Design review of the part built by this model. Coordinates are the model's own, in mm. Face numbers are marked on the shaded views. A direction names the side the tool comes from. Coordinates: 2 decimals unless noted, no trailing zeros. Loops run counter-clockwise (first coordinate to the right, second up) from the corner with the lowest first, then second, coordinate; pieces in that order, holes last. Notation, with made-up numbers: M 21.25,16.25 L 43.25,16.25 A23 cw 43.25,29.25 Z; hole C 22.25,-20.75 d8. An arc over 180 degrees is marked long. One line per item, written item: value.
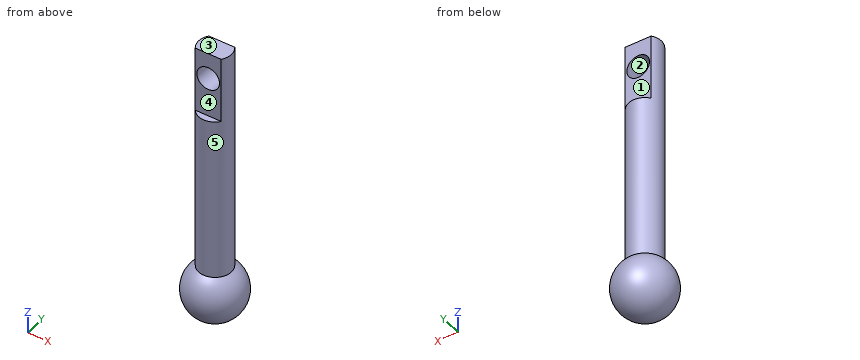
```python
from build123d import *

# Parameters (mm, degrees)
CUT_EXTRUDE3_START      = -10
CUT_EXTRUDE3_DEPTH      = 10
CUT_EXTRUDE4_DEPTH      = 44.707447118
CUT_EXTRUDE4_DEPTH_BACK = 44.707447118
SKETCH4_R               = 1.75


with BuildPart() as part:
    # Sketch1 → Revolve1 (revolve)
    with BuildSketch(Plane(origin=(0, 0, 0), x_dir=(1, 0, 0), z_dir=(0, 1, 0)), mode=Mode.PRIVATE) as revolve1_sk:
        with BuildLine():
            Line((0, 43.241657387), (0, 0))
            Line((0, 0), (2.5, 0))
            Line((2.5, 0), (2.5, 35))
            ThreePointArc((2.5, 35), (4.30624304, 40.047900427), (0, 43.241657387))
        make_face()
    revolve(revolve1_sk.sketch.rotate(Axis((0, 0, -43.241657387), (0, 0, 1)), 180), axis=Axis((0, 0, -43.241657387), (0, 0, 1)))

    # Sketch2 → Cut-Extrude3 (cut)
    with BuildSketch(Plane.XY.offset(CUT_EXTRUDE3_START)):
        with BuildLine():
            ThreePointArc((2, 1.5), (0, 2.5), (-2, 1.5))
            Line((-2, 1.5), (2, 1.5))
        make_face()
        with BuildLine():
            Line((2, -1.5), (-2, -1.5))
            ThreePointArc((-2, -1.5), (0, -2.5), (2, -1.5))
        make_face()
    extrude(amount=CUT_EXTRUDE3_DEPTH, mode=Mode.SUBTRACT)

    # Sketch4 → Cut-Extrude4 (cut, two sides: drawn at the far end of the back side and taken through both)
    with BuildSketch(Plane(origin=(0, 0, 0), x_dir=(1, 0, 0), z_dir=(0, 1, 0)).offset(-CUT_EXTRUDE4_DEPTH_BACK)):
        with Locations(Location((0, 4, 0), (0, 0, 90))):
            Circle(SKETCH4_R)
    extrude(amount=CUT_EXTRUDE4_DEPTH + CUT_EXTRUDE4_DEPTH_BACK, mode=Mode.SUBTRACT)


solid = part.part
```
(1) We need section D-D on z = -26. State the section outline as (x, y) points, then the cut area to 3 significant figures.
Reply:
outline: C 0,0 d5
area: 19.6 mm2
(2) We need section B-B on y = 0. State the section outline as (x, z) points, then the cut area to 3 significant figures.
Reply:
outline: M -2.5,-35 A4.5 ccw long 2.5,-35 L 2.5,0 L -2.5,0 Z; hole C 0,-4 d3.5
area: 226 mm2
(3) Insertion check: pin 1 (1 mm diameter, centred on x = -2, y = -2.5, fed in from -Z); pin 2 (5 mm diameter, centred on x = 3, z = -17, fed in from -Y); pin 3 (5 mm diameter, centred on x = -1.5, z = -28, fed in from +Y). Each pin has a flat end and moves straight along its axis. Give the tip position at first contact, or say it passes through.
Reply:
pin 1: stops at z = -42.34
pin 2: stops at y = -2.45
pin 3: stops at y = 2.5
(4) Tool access review of the marked faces 4 and 5: name each direction out of +Z, -Z, +X, -X, +Y, -Y from which nothing blocks a thin tool from reaching the whole face with its end or side.
Reply:
face 4: +Z, +X, -X, -Y
face 5: +Z
(5) We need section A-A on z = -4. State the section outline as (x, y) points.
Reply:
outline: M -2,-1.5 L -1.75,-1.5 L -1.75,1.5 L -2,1.5 A2.5 ccw Z; M 1.75,-1.5 L 2,-1.5 A2.5 ccw 2,1.5 L 1.75,1.5 Z
(6) Mouldability with a two-part tool opening along Z and no side actions: class the marked faces 1, 2 and 3 as released by +Z, released by -Z, zero draft, split by the parting line, or undercut.
Reply:
face 1: zero draft
face 2: undercut
face 3: released by +Z
(7) To check wall thickness, follow line 1 along X through (y, z) = (0.1, -4); line 2 along Y through (x, z) = (-0.5, -1.5); line 3 along Z through (x, y) = (0.25, 0). State the ranges of each line that lie inside material, in increasing order. Write a range as [from, to].
Reply:
line 1: x = [-2.5, -1.75], [1.75, 2.5]
line 2: y = [-1.5, 1.5]
line 3: z = [-43.23, -5.73], [-2.27, 0]
(8) We need section C-C on x = 0. State the section outline as (y, z) points, then the cut area to 3 significant figures.
Reply:
outline: M -2.5,-35 A4.5 ccw long 2.5,-35 L 2.5,-10 L 1.5,-10 L 1.5,-5.75 L -1.5,-5.75 L -1.5,-10 L -2.5,-10 Z; M -1.5,-2.25 L 1.5,-2.25 L 1.5,0 L -1.5,0 Z
area: 206 mm2
